For this review, take the finished solid that the model builds, in its own axes (mm). Face numbers are marked on the shaded views. Coordinates: 2 decimals unless noted, no trailing zeros. Write each loop counter-clockwise with the first axis right and the second up, starting at its lowest first coordinate (ties: lowest second). Pieces come first, ordered by that corner, then holes. Notation, with made-up numbers: (65.25, 4) - (73.25, 4) arc R24 cw to (73.25, 22) - close; hole circle Ø7 at (58.25, 0.5). An arc over 180 degrees is marked (long way). Write each question's results on one line, items separated by ' | '.
from build123d import *

# Parameters (mm, degrees)
SKETCH_W    = 60
SKETCH_H    = 41
SKETCH_R    = 2.5
SKETCH_R_2  = 6.5
PAD_DEPTH   = 10
FILLET_R    = 10
FILLET001_R = 1


with BuildPart() as part:
    # Sketch → Pad (new body)
    with BuildSketch(Plane.XY):
        with Locations((5, -94.5)):
            Rectangle(SKETCH_W, SKETCH_H)
        with Locations((25, -80)):
            Circle(SKETCH_R, mode=Mode.SUBTRACT)
        with Locations((-18, -80)):
            Circle(SKETCH_R, mode=Mode.SUBTRACT)
        with Locations((0, -85)):
            Circle(SKETCH_R_2, mode=Mode.SUBTRACT)
    extrude(amount=PAD_DEPTH)

    # Fillet
    fillet_edges = [part.edges().sort_by_distance(p)[0] for p in [
        (-25, -115, 5),
        (35, -115, 5),
    ]]
    fillet(fillet_edges, radius=FILLET_R)

    # Fillet001
    fillet001_edges = [part.edges().sort_by_distance(p)[0] for p in [
        (-25, -74, 5),
        (35, -74, 5),
    ]]
    fillet(fillet001_edges, radius=FILLET001_R)


solid = part.part
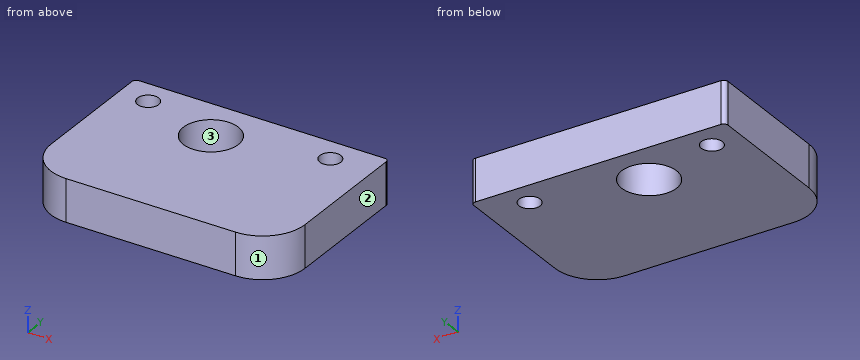
Q1. Mouldability with a two-part tool opening along Y and no side actions: class the marked faces 1, 2 and 3 as pulls with the +Y half, pulls with the -Y half, needs draft (parallel to the pull), parting line crosses it, or undercut.
Results found:
face 1: pulls with the -Y half | face 2: needs draft | face 3: undercut
Q2. Take a section at C-C on y = -80. State the section outline as (x, z) points, plus the area to 3 significant figures.
Results found:
outline: (-25, 0) - (-20.5, 0) - (-20.5, 10) - (-25, 10) - close; (-15.5, 0) - (-4.15, 0) - (-4.15, 10) - (-15.5, 10) - close; (4.15, 0) - (22.5, 0) - (22.5, 10) - (4.15, 10) - close; (27.5, 0) - (35, 0) - (35, 10) - (27.5, 10) - close | area: 417 mm2
Q3. Take a section at B-B on y = -85. State the section outline as (x, z) points.
Results found:
outline: (-25, 0) - (-6.5, 0) - (-6.5, 10) - (-25, 10) - close; (6.5, 0) - (35, 0) - (35, 10) - (6.5, 10) - close
Q4. Take a section at A-A on z = 1.25. State the section outline as (x, y) points, plus the area to 3 significant figures.
Results found:
outline: (-25, -105) arc R10 ccw to (-15, -115) - (25, -115) arc R10 ccw to (35, -105) - (35, -75) arc R1 ccw to (34, -74) - (-24, -74) arc R1 ccw to (-25, -75) - close; hole circle Ø5 at (-18, -80); hole circle Ø13 at (0, -85); hole circle Ø5 at (25, -80) | area: 2,240 mm2
Q5. Wall thickness on line 1 along Y through (x, z) = (0, 4); line 2 along Y through (x, z) = (25, 5.25); line 3 along X through (y, z) = (-88, 9.5): over which ranges is each line inside the solid? List them lowest first. Write a range as from..to.
Results found:
line 1: -115..-91.5, -78.5..-74 | line 2: -115..-82.5, -77.5..-74 | line 3: -25..-5.77, 5.77..35
Q6. Take a section at D-D on x = -18. State the section outline as (y, z) points, plus the area to 3 significant figures.
Results found:
outline: (-114.54, 0) - (-82.5, 0) - (-82.5, 10) - (-114.54, 10) - close; (-77.5, 0) - (-74, 0) - (-74, 10) - (-77.5, 10) - close | area: 355 mm2
Q7. For pin 1 (4.5 mm diameter, centred on x = 25, y = -80, fed in from +Z); pin 2 (2 mm diameter, centred on y = -108, z = 8, fed in from +X), all flat-tipped, find the tip position at first contact; note any pin that passes through.
Results found:
pin 1: through | pin 2: x = 34.8
